from build123d import *

# Parameters (mm, degrees)
BOSS_EXTRUDE1_DEPTH = 300
SKETCH2_R           = 6
BOSS_EXTRUDE2_DEPTH = 20


with BuildPart() as part:
    # Sketch1 → Boss-Extrude1 (new body)
    with BuildSketch(Plane.XY):
        with BuildLine():
            Line((-233.856725658, -45.403733341), (-191.664199257, -10))
            Line((-191.664199257, -10), (-500, -10))
            Line((-500, -10), (-500, 10))
            Line((-500, 10), (500, 10))
            Line((500, 10), (500, -10))
            Line((500, -10), (191.664199257, -10))
            Line((191.664199257, -10), (233.856725658, -45.403733341))
            ThreePointArc((233.856725658, -45.403733341), (234.596266659, -53.856725658), (226.143274342, -54.596266659))
            Line((226.143274342, -54.596266659), (172.995513335, -10))
            Line((172.995513335, -10), (-172.995513335, -10))
            Line((-172.995513335, -10), (-226.143274342, -54.596266659))
            ThreePointArc((-226.143274342, -54.596266659), (-234.596266659, -53.856725658), (-233.856725658, -45.403733341))
        make_face()
    extrude(amount=BOSS_EXTRUDE1_DEPTH)

    # Sketch2 → Boss-Extrude2 (add)
    with BuildSketch(Plane.XY.offset(300)):
        with Locations((-230, -50)):
            Circle(SKETCH2_R)
        with Locations((230, -50)):
            Circle(SKETCH2_R)
    extrude(amount=BOSS_EXTRUDE2_DEPTH)


solid = part.part
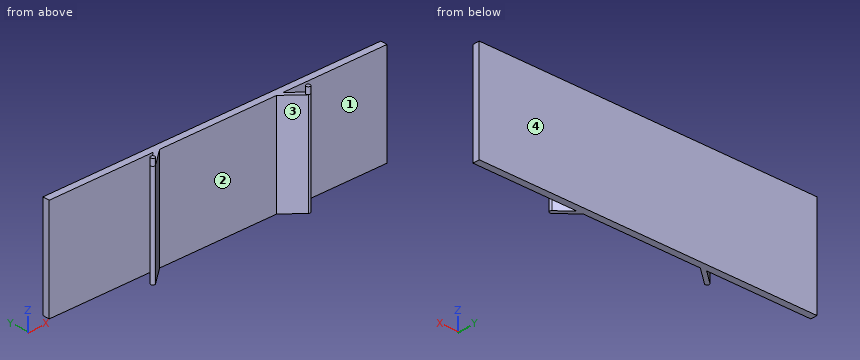
Design review of the part built by this model. Coordinates are the model's own, in mm. Face numbers are marked on the shaded views. A direction names the side the tool comes from. Coordinates: 2 decimals unless noted, no trailing zeros. Order: outer loops, then holes, each group sorted by start corner. A loop starts at its lowest first (then second) coordinate and runs counter-clockwise, first axis right, second up. Notation, with made-up numbers: M -21.5,59.5 L 26.5,59.5 A27 cw 26.5,89.5 Z; hole C -17.5,85.5 d1. An arc over 180 degrees is marked long. Use a Markdown table: item, result.
(1) For the marked faces 3 and 4, list the 3-axis set-ups (+Z, -Z, +X, -X, +Y, -Y) from which the entire face can be reached by the end or side of a thin tool; tool diameter is ignored.
Worked answers:
| item | result |
|---|---|
| face 3 | +Z, -Z, -Y |
| face 4 | +Z, -Z, +X, -X, +Y |
(2) Add section A-A (z = 36). Give the boundary of the cut face in (x, y).
Worked answers:
| item | result |
|---|---|
| outline | M -500,-10 L -191.66,-10 L -233.86,-45.4 A6 ccw -226.14,-54.6 L -173,-10 L 173,-10 L 226.14,-54.6 A6 ccw 233.86,-45.4 L 191.66,-10 L 500,-10 L 500,10 L -500,10 Z |
(3) Add section C-C (x = -162). Give the boundary of the cut face in (y, z).
Worked answers:
| item | result |
|---|---|
| outline | M -10,0 L 10,0 L 10,300 L -10,300 Z |
(4) Wall thickness on probe 1 along Y at (x, z) = (-332, 121); probe 2 along X at (y, z) = (-41.5, 296); probe 3 along X at (y, z) = (-33, 16): over which ranges is each line inside the solid? List them lowest first.
Worked answers:
| item | result |
|---|---|
| probe 1 | y = -10 to 10 |
| probe 2 | x = -229.2 to -210.54, 210.54 to 229.2 |
| probe 3 | x = -219.07 to -200.41, 200.41 to 219.07 |
(5) Add section B-B (y = -28). Give the boundary of the cut face in (x, z), then the cut area to 3 significant figures.
Worked answers:
| item | result |
|---|---|
| outline | M -213.12,0 L -194.45,0 L -194.45,300 L -213.12,300 Z; M 194.45,0 L 213.12,0 L 213.12,300 L 194.45,300 Z |
| area | 11,200 mm2 |
(6) For P1, Ø1, axis at y = -24.5, z = 206, coming from the -X side; P2, Ø3, axis at x = 153, z = 235.5, coming from the -Y side; P3, Ø6, axis at y = -16.5, z = 182.5, coming from the -X side; P4, Ø3, axis at x = -347, y = -12, coming from the -Z side, all flat-tipped, find the tip position at first contact; note any pin that passes through.
Worked answers:
| item | result |
|---|---|
| P1 | stops at x = -209.54 |
| P2 | stops at y = -10 |
| P3 | stops at x = -202.99 |
| P4 | passes through |
(7) Draft analysis for pull direction X (two halves, no side actions). For the marked faces 1 and 2, state which applies: released by +X, released by -X, zero draft, split by the parting line, or undercut.
Worked answers:
| item | result |
|---|---|
| face 1 | zero draft |
| face 2 | undercut |
